Check sheet for the modelled part. Datum: model origin and axes. Units: mm. A direction names the side the tool comes from. Round coordinates to 2 decimals unless told otherwise and drop trailing zeros. Loops run counter-clockwise (first coordinate to the right, second up) from the corner with the lowest first, then second, coordinate; pieces in that order, holes last. Notation, with made-up numbers: (72, 68.5) - (131, 68.5) arc R21 ccw to (131, 87.5) - close; hole circle Ø8 at (66, 89.25). An arc over 180 degrees is marked (long way). Put each result on its own line as item: value. Start each with the question number.
Autodesk Inventor part; units mm, degrees
ref_plane "YZ Plane" through (0, 0, 0) normal (1, 0, 0) x (0, 1, 0)
ref_plane "XZ Plane" through (0, 0, 0) normal (0, 1, 0) x (-1, 0, 0)
ref_plane "XY Plane" through (0, 0, 0) normal (0, 0, 1) x (1, 0, 0)
sketch "Sketch1" plane through (0, 0, 0) normal (0, 0, 1) x (1, 0, 0)
  line L0 (-14.1, -14.1) -> (14.1, -14.1)
  line L1 (14.1, -14.1) -> (14.1, 14.1)
  line L2 (14.1, 14.1) -> (-14.1, 14.1)
  line L3 (-14.1, 14.1) -> (-14.1, -14.1)
  line L4 (-14.1, -14.1) -> (14.1, 14.1) construction
  line L5 (14.1, -14.1) -> (-14.1, 14.1) construction
  point P0 (0, 0)
  dimension "d0" = 28.2
  dimension "d1" = 28.2
extrude "Extrusion1" add sketch "Sketch1" along normal blind 32
sketch "Sketch2" plane through (0, 0, 32) normal (0, 0, 1) x (1, 0, 0)
  line L0 (-11.5, -11.5) -> (11.5, -11.5) construction
  line L1 (11.5, -11.5) -> (11.5, 11.5) construction
  line L2 (11.5, 11.5) -> (-11.5, 11.5) construction
  line L3 (-11.5, 11.5) -> (-11.5, -11.5) construction
  line L4 (-11.5, -11.5) -> (11.5, 11.5) construction
  line L5 (11.5, -11.5) -> (-11.5, 11.5) construction
  circle A0 centre (-11.5, 11.5) radius 1.25
  line L6 (11.5, -11.5) -> (11.5, 11.5) construction
  line L7 (11.5, 11.5) -> (-11.5, 11.5) construction
  line L8 (-11.5, 11.5) -> (-11.5, -11.5) construction
  line L9 (-11.5, -11.5) -> (11.5, -11.5) construction
  line L10 (11.5, -11.5) -> (-11.5, 11.5) construction
  line L11 (11.5, 11.5) -> (-11.5, -11.5) construction
  circle A1 centre (-11.5, -11.5) radius 1.25
  line L12 (11.5, 11.5) -> (-11.5, 11.5) construction
  line L13 (-11.5, 11.5) -> (-11.5, -11.5) construction
  line L14 (-11.5, -11.5) -> (11.5, -11.5) construction
  line L15 (11.5, -11.5) -> (11.5, 11.5) construction
  line L16 (11.5, 11.5) -> (-11.5, -11.5) construction
  line L17 (-11.5, 11.5) -> (11.5, -11.5) construction
  circle A2 centre (11.5, -11.5) radius 1.25
  line L18 (-11.5, 11.5) -> (-11.5, -11.5) construction
  line L19 (-11.5, -11.5) -> (11.5, -11.5) construction
  line L20 (11.5, -11.5) -> (11.5, 11.5) construction
  line L21 (11.5, 11.5) -> (-11.5, 11.5) construction
  line L22 (-11.5, 11.5) -> (11.5, -11.5) construction
  line L23 (-11.5, -11.5) -> (11.5, 11.5) construction
  circle A3 centre (11.5, 11.5) radius 1.25
  point P0 (0, 0)
  point P1 (0, 0)
  point P2 (0, 0)
  point P3 (0, 0)
  dimension "d4" = 23
  dimension "d5" = 23
  dimension "d6" = 2.5
  dimension "d9" = 360
extrude "Extrusion2" cut sketch "Sketch2" against normal blind 4.5
sketch "Sketch3" plane through (0, 0, 32) normal (0, 0, 1) x (1, 0, 0)
  circle A0 centre (0, 0) radius 11
  dimension "d13" = 22
extrude "Extrusion3" add sketch "Sketch3" along normal blind 2
sketch "Sketch4" plane through (0, 0, 34) normal (0, 0, 1) x (1, 0, 0)
  circle A0 centre (0, 0) radius 2.5
  dimension "d16" = 5
extrude "Extrusion4" add sketch "Sketch4" along normal blind 18
fillet "Fillet1" radius 2 4 edges at (-14.1, 14.1, 16) (14.1, 14.1, 16) (14.1, -14.1, 16) (-14.1, -14.1, 16)
chamfer "Chamfer1" distance 0.5 angle 45 1 edges at (-2.5, 0, 52)
chamfer "Chamfer2" distance 0.5 angle 45 1 edges at (-11, 0, 34)
sketch "Sketch5" plane through (14.1, -12.1, 0) normal (1, 0, 0) x (0, 0, -1)
  line L0 (0, 12.1) -> (-5, 12.1) construction
  line L1 (-7, 7.1) -> (-3, 7.1)
  line L2 (-3, 7.1) -> (-3, 17.1)
  line L3 (-3, 17.1) -> (-7, 17.1)
  line L4 (-7, 17.1) -> (-7, 7.1)
  line L5 (-7, 7.1) -> (-3, 17.1) construction
  line L6 (-3, 7.1) -> (-7, 17.1) construction
  dimension "d26" = 5
  dimension "d27" = 4
  dimension "d28" = 10
extrude "Extrusion5" add sketch "Sketch5" along normal blind 5
properties part number "nema11_SY28STH32-0674A"
Q1. Cross-section at D-D on z = 44. Enter the section's corners in (x, y), and give its area (3 significant figures).
Q2. Cross-section at B-B on x = 0. Enter the section's corners in (y, z), and give its area (3 significant figures).
Q3. Depth check by flat-ended pin: pin 1 Ø4.5 at (x, z) = (17, 4) entering from -Y; pin 2 Ø2 at (x, y) = (11.5, -11.5) entering from +Z; pin 3 Ø2 at (x, y) = (-11.5, 11.5) entering from -Z; pin 4 Ø3 at (x, y) = (-11.5, -12) entering from +Z. Enter the tip coordinate at first touch or a pass-through.
Q4. Set-up check for faces 1 (the face through (17, -5, 5)), 2 (the face through (17, 0, 3)), 3 (the face through (-2.38, 10.74, 32.74)): record each of +Z, -Z, +X, -X, +Y, -Y from which the full face is reachable in a straight line by a thin tool's end or side.
Q5. Cross-section at A-A on y = 0. Enter the section's corners in (x, z), and give its area (3 significant figures).
Q6. Draft check along X on faces 4 (the face through (0, 14.1, 16)), 5 (the face through (19.1, 0, 5)), 6 (the face through (11, -11, 27.5)). Enter one of: +X half, -X half, draft (parallel to the pull), parting line (faces both ways), or undercut.
Q7. Cross-section at C-C on z = 23. Enter the section's corners in (x, y).
Q8. Material ranges on line 1 (Y direction, x = -11.5, z = 31); line 2 (Z direction, x = 4, y = 2); line 3 (Y direction, x = -11, z = 30), recorded low to high. Write a range as from..to.
Answer list:
1. outline: circle Ø5 at (0, 0)
1. area: 19.6 mm2
2. outline: (-14.1, 0) - (14.1, 0) - (14.1, 32) - (11, 32) - (11, 33.5) - (10.5, 34) - (2.5, 34) - (2.5, 51.5) - (2, 52) - (-2, 52) - (-2.5, 51.5) - (-2.5, 34) - (-10.5, 34) - (-11, 33.5) - (-11, 32) - (-14.1, 32) - close
2. area: 1,040 mm2
3. pin 1: stops at y = -5
3. pin 2: stops at z = 27.5
3. pin 3: stops at z = 0
3. pin 4: stops at z = 32
4. face 1: +Z, -Z, +X, -Y
4. face 2: -Z, +X, +Y, -Y
4. face 3: +Z
5. outline: (-14.1, 0) - (14.1, 0) - (14.1, 3) - (19.1, 3) - (19.1, 7) - (14.1, 7) - (14.1, 32) - (11, 32) - (11, 33.5) - (10.5, 34) - (2.5, 34) - (2.5, 51.5) - (2, 52) - (-2, 52) - (-2.5, 51.5) - (-2.5, 34) - (-10.5, 34) - (-11, 33.5) - (-11, 32) - (-14.1, 32) - close
5. area: 1,060 mm2
6. face 4: draft
6. face 5: +X half
6. face 6: undercut
7. outline: (-14.1, -12.1) arc R2 ccw to (-12.1, -14.1) - (12.1, -14.1) arc R2 ccw to (14.1, -12.1) - (14.1, 12.1) arc R2 ccw to (12.1, 14.1) - (-12.1, 14.1) arc R2 ccw to (-14.1, 12.1) - close
8. line 1: y = -14.1..-12.75, -10.25..10.25, 12.75..14.1
8. line 2: z = 0..34
8. line 3: y = -14.1..-12.65, -10.35..10.35, 12.65..14.1
